```python
from build123d import *

# Parameters (mm, degrees)
SKETCH_1_W                      = 40
SKETCH_1_H                      = 51.65
EXTRUDE_1_DEPTH                 = 12
SHELL_1_T                       = -2
SKETCH_3_W                      = 3.9
SKETCH_3_H                      = 21.85
SKETCH_3_W_2                    = 4.4
SKETCH_3_H_2                    = 2
EXTRUDE_6_DEPTH                 = 10
CUT_EXTRUDE_1_REACH             = 58.672
SKETCH_4_R                      = 1.1
SKETCH_4_R_2                    = 1.6
SKETCH_4_W                      = 10
SKETCH_4_H                      = 4.5
CUT_EXTRUDE_1_DIRECTION_2_DEPTH = 57.672061018
CUT_EXTRUDE_START               = -19.3
SKETCH_6_R                      = 1.1
SKETCH_6_R_2                    = 1.6
CUT_EXTRUDE_4_DEPTH             = 19.3


with BuildPart() as part:
    # 草图1 → 凸台-拉伸1 (new body)
    with BuildSketch(Plane(origin=(0, 0, 0), x_dir=(0, 0, -1), z_dir=(1, 0, 0))):
        Rectangle(SKETCH_1_W, SKETCH_1_H)
    extrude(amount=EXTRUDE_1_DEPTH)

    # 抽壳1
    shell_1_openings = [part.faces().sort_by_distance(p)[0] for p in [
        (12, 0, 0),
    ]]
    offset(amount=SHELL_1_T, openings=shell_1_openings, kind=Kind.INTERSECTION)

    # 草图3 → 凸台-拉伸6 (add)
    # profile 1 of 2: a face of its own
    with BuildSketch(Plane(origin=(2, 0, 0), x_dir=(0, 0, -1), z_dir=(1, 0, 0))):
        Polygon((2.9, -8.525), (-5, -8.525), (-5, 23.825), (-3, 23.825), (-3, 17.325), (2.9, 17.325), (2.9, -3.575), (7.4, -3.575), (7.4, -5.575), (2.9, -5.575), align=None)
        with Locations((-1.05, 4.4)):
            Rectangle(SKETCH_3_W, SKETCH_3_H, mode=Mode.SUBTRACT)
    # profile 2 of 2: a face of its own
    with BuildSketch(Plane(origin=(2, 0, 0), x_dir=(0, 0, -1), z_dir=(1, 0, 0))):
        with Locations((15.8, -4.575)):
            Rectangle(SKETCH_3_W_2, SKETCH_3_H_2)
    extrude(amount=EXTRUDE_6_DEPTH)

    # 草图4 → 切除-拉伸1 (cut, up to next)
    with BuildSketch(Plane(origin=(0, 25.825, 0), x_dir=(1, 0, 0), z_dir=(0, 1, 0)), mode=Mode.PRIVATE) as cut_extrude_1_sk1:
        with Locations((12, 10.5)):
            Circle(SKETCH_4_R)
    cut_extrude_1_tool1 = extrude(cut_extrude_1_sk1.sketch, amount=-CUT_EXTRUDE_1_REACH, mode=Mode.PRIVATE) & part.part
    # 草图4 → 切除-拉伸1 (cut, up to next)
    with BuildSketch(Plane(origin=(0, 25.825, 0), x_dir=(1, 0, 0), z_dir=(0, 1, 0)), mode=Mode.PRIVATE) as cut_extrude_1_sk2:
        with Locations((12, -9.5)):
            Circle(SKETCH_4_R_2)
    cut_extrude_1_tool2 = extrude(cut_extrude_1_sk2.sketch, amount=-CUT_EXTRUDE_1_REACH, mode=Mode.PRIVATE) & part.part
    # 草图4 → 切除-拉伸1 (cut, up to next)
    with BuildSketch(Plane(origin=(0, 25.825, 0), x_dir=(1, 0, 0), z_dir=(0, 1, 0)), mode=Mode.PRIVATE) as cut_extrude_1_sk3:
        with Locations((7, 1.25)):
            Rectangle(SKETCH_4_W, SKETCH_4_H)
    cut_extrude_1_tool3 = extrude(cut_extrude_1_sk3.sketch, amount=-CUT_EXTRUDE_1_REACH, mode=Mode.PRIVATE) & part.part
    add(cut_extrude_1_tool1.solids().sort_by_distance((12, 25.825, -10.5))[0], mode=Mode.SUBTRACT)
    add(cut_extrude_1_tool2.solids().sort_by_distance((12, 25.825, 9.5))[0], mode=Mode.SUBTRACT)
    add(cut_extrude_1_tool3.solids().sort_by_distance((7, 25.825, -1.25))[0], mode=Mode.SUBTRACT)

    # 草图4 → 切除-拉伸1 direction 2 (cut)
    with BuildSketch(Plane(origin=(0, 25.825, 0), x_dir=(1, 0, 0), z_dir=(0, 1, 0))):
        with Locations((12, 10.5)):
            Circle(SKETCH_4_R)
        with Locations((12, -9.5)):
            Circle(SKETCH_4_R_2)
        with Locations((7, 1.25)):
            Rectangle(SKETCH_4_W, SKETCH_4_H)
    extrude(amount=CUT_EXTRUDE_1_DIRECTION_2_DEPTH, mode=Mode.SUBTRACT)

    # 草图6 → 切除-拉伸4 (cut)
    with BuildSketch(Plane.XZ.offset(25.825).offset(CUT_EXTRUDE_START)):
        with Locations((12, -0.5)):
            Circle(SKETCH_6_R)
        with Locations((12, 9.5)):
            Circle(SKETCH_6_R_2)
    extrude(amount=CUT_EXTRUDE_4_DEPTH, mode=Mode.SUBTRACT)


solid = part.part
```
Here's how the part is built. I have some questions about the finished solid (model axes, mm). A direction names the side the tool comes from. Round coordinates to 2 decimals unless told otherwise and drop trailing zeros. Write each loop counter-clockwise with the first axis right and the second up, starting at its lowest first coordinate (ties: lowest second). Pieces come first, ordered by that corner, then holes.
Q1. If we section it at A-A on y = -21.5: Write out the boundary of the cut face in (x, z).
Q2. Will this pin go through, and if not, where does the flat tip stop? P1, Ø3, axis at y = 8, z = 1, coming from the +X side.
Q3. If we section it at C-C on z = 9.5: Write out the boundary of the cut face in (x, y) (3 decimals), plus the area to 3 significant figures.
Q4. Which directions (+Z, -Z, +X, -X, +Y, -Y) give clear straight access to the entire face, cutting with the end or side of a thin tool? Please do faces 4 (the flat face through (12, -25, 4)), 5 (the flat face through (7, 7, -2.9)), 6 (the flat face through (7, -3.575, -16)).
Q5. If we mould it in two halves opening along Z, with no side actions, what happens to faces 1 (the flat face through (6, 25.825, -4)), 2 (the flat face through (6, 0, 20)), 3 (the flat face through (7, 7, 5))? For each: +Z half, -Z half, draft (parallel to the pull), parting line (faces both ways), or undercut.
Q6. If we section it at D-D on y = 19: Write out the boundary of the cut face in (x, z), plus the area to 3 significant figures.
Q7. Please list where these lines run through material, in increasing order: probe 1 along Y at (x, z) = (2.5, 2) (3 decimals); probe 2 along Z at (x, y) = (10, 4); probe 3 along Y at (x, z) = (3.5, -2) (3 decimals).
Answer below:
1. outline: (0, -20) - (12, -20) - (12, -18) - (2, -18) - (2, 18) - (12, 18) - (12, 20) - (0, 20) - close
2. P1: stops at x = 2
3. outline: (0, -25.825) - (10.4, -25.825) - (10.4, -23.825) - (2, -23.825) - (2, 23.825) - (10.4, 23.825) - (10.4, 25.825) - (0, 25.825) - close
3. area: 137 mm2
4. face 4: +Z, -Z, +X, +Y, -Y
4. face 5: +X, +Y
4. face 6: +X
5. face 1: draft
5. face 2: +Z half
5. face 3: undercut
6. outline: (0, -20) - (12, -20) - (12, -18) - (2, -18) - (2, 3) - (12, 3) - (12, 5) - (2, 5) - (2, 18) - (12, 18) - (12, 20) - (0, 20) - close
6. area: 140 mm2
7. probe 1: y = -25.825 to -23.825, -8.525 to -6.525, 15.325 to 17.325, 23.825 to 25.825
7. probe 2: z = -20 to -18, -2.9 to -0.9, 3 to 5, 18 to 20
7. probe 3: y = -25.825 to -23.825, -8.525 to 17.325
